The listing builds one solid part. Answer for the finished solid, in the listing's coordinates (mm). A direction names the side the tool comes from. Round coordinates to 2 decimals unless told otherwise and drop trailing zeros. Order: outer loops, then holes, each group sorted by start corner. A loop starts at its lowest first (then second) coordinate and runs counter-clockwise, first axis right, second up. Notation, with made-up numbers: M -6.75,77.25 L 6.25,77.25 A19 cw 6.25,100.25 Z; hole C 62.25,52.5 d5. An arc over 180 degrees is marked long. Write item = value, one per line. Start each with the question number.
(1) Which of the six approach directions +Z, -Z, +X, -X, +Y, -Y give full straight-line access (tool end or side, diameter ignored) to faces 1 (the face through (7.45, 0, -43)), 2 (the face through (8.72, -0.1, 51.9)), 3 (the face through (10.7, 0, 37)), 4 (the face through (6.7, 0, -46)), 5 (the face through (-4.3, 0, 37))?
(2) Each of these flat-tipped pins is pushed along its axis until it touches: pin 1 (4.5 mm diameter, centred on y = 3, z = -43.5, fed in from +X); pin 2 (3 mm diameter, centred on x = 9, y = -0.5, fed in from +Z); pin 3 (0.9 mm diameter, centred on y = 3, z = 55.5, fed in from +X); pin 4 (1.5 mm diameter, centred on x = 1.5, z = -36, fed in from -Y). Where does it stop, or does it pass through?
(3) A cutting plane is placed at B-B, the plane z = -0.5. Determine the outline of the cut face in (x, y), and give its area (3 significant figures).
(4) For a pull along Z with two mould halves and no side action, classify faces 6 (the face through (12.55, -0.1, 43.48)), 7 (the face through (-6.4, 0.1, -8.5)), 8 (the face through (10.2, 0, -43)) as released by +Z, released by -Z, zero draft, split by the parting line, or undercut.
(5) A cutting plane is placed at A-A, the plane x = 3.5. Determine the outline of the cut face in (y, z) (3 decimals).
(6) A cutting plane is placed at C-C, the plane x = -1.25. Determine the outline of the cut face in (y, z) (3 decimals).
(7) Straight lines are drawn through the part: probe 1 along Z at (x, y) = (3.25, -0.75) (3 decimals); probe 2 along X at (y, z) = (5.25, -1); probe 3 along X at (y, z) = (-4, -40). For each, find the intervals that lie inside material, in ascending order. Write a range as from..to.
from build123d import *

# Parameters (mm, degrees)
F1_DEPTH = 7.45
F2_W     = 9.95
F2_H     = 59.4720471648
F3_DEPTH = 14.901
F5_DEPTH = 14.9


with BuildPart() as f1:
    # F0 (on Front) → F1 (new body, symmetric)
    with BuildSketch(Plane.XZ):
        with BuildLine():
            Line((-8.5, -30.0970471648), (-4.3, -36.825))
            Line((-4.3, -36.825), (-4.3, -40.625))
            ThreePointArc((-4.3, -40.625), (-4.0071067812, -41.3321067812), (-3.3, -41.625))
            Line((-3.3, -41.625), (7.45, -41.625))
            Line((7.45, -41.625), (7.45, -44.825))
            Line((7.45, -44.825), (6.7, -44.825))
            Line((6.7, -44.825), (6.7, -47.025))
            Line((6.7, -47.025), (10.2, -47.025))
            Line((10.2, -47.025), (10.2, -38.425))
            ThreePointArc((10.2, -38.425), (9.9071067812, -37.7178932188), (9.2, -37.425))
            Line((9.2, -37.425), (0, -37.425))
            Line((0, -37.425), (0, 37.425))
            Line((0, 37.425), (8.4, 37.425))
            Line((8.4, 37.425), (8.4, 33.425))
            ThreePointArc((8.4, 33.425), (8.6928932188, 32.7178932188), (9.4, 32.425))
            Line((9.4, 32.425), (9.7, 32.425))
            ThreePointArc((9.7, 32.425), (10.4071067812, 32.7178932188), (10.7, 33.425))
            Line((10.7, 33.425), (10.7, 40.875))
            Line((10.7, 40.875), (12.0584372697, 42.3947607825))
            ThreePointArc((12.0584372697, 42.3947607825), (12.5542284753, 43.4993517405), (12.3218441058, 44.6875973417))
            Line((12.3218441058, 44.6875973417), (9.6272657122, 49.6124442137))
            ThreePointArc((9.6272657122, 49.6124442137), (8.7116734449, 51.9351925206), (8.4, 54.4123539124))
            Line((8.4, 54.4123539124), (8.4, 57.375))
            ThreePointArc((8.4, 57.375), (8.1071067812, 58.0821067812), (7.4, 58.375))
            Line((7.4, 58.375), (7.1, 58.375))
            ThreePointArc((7.1, 58.375), (6.3928932188, 58.0821067812), (6.1, 57.375))
            Line((6.1, 57.375), (6.1, 54.4123539124))
            ThreePointArc((6.1, 54.4123539124), (6.4116734449, 51.9351925206), (7.3272657122, 49.6124442137))
            Line((7.3272657122, 49.6124442137), (10.0218441058, 44.6875973417))
            ThreePointArc((10.0218441058, 44.6875973417), (10.2542284753, 43.4993517405), (9.7584372697, 42.3947607825))
            Line((9.7584372697, 42.3947607825), (8.4, 40.875))
            Line((8.4, 40.875), (-3.3, 40.875))
            ThreePointArc((-3.3, 40.875), (-4.0071067812, 40.5821067812), (-4.3, 39.875))
            Line((-4.3, 39.875), (-4.3, 33.875))
            Line((-4.3, 33.875), (-8.5, 29.375))
            Line((-8.5, 29.375), (-8.5, 20.075))
            Line((-8.5, 20.075), (-13.95, 20.075))
            Line((-13.95, 20.075), (-13.95, 29.375))
            Line((-13.95, 29.375), (-16.45, 29.375))
            ThreePointArc((-16.45, 29.375), (-17.8642135624, 28.7892135624), (-18.45, 27.375))
            Line((-18.45, 27.375), (-18.45, 13.875))
            Line((-18.45, 13.875), (-8.5, 6.6029528352))
            Line((-8.5, 6.6029528352), (-8.5, -30.0970471648))
        make_face()
    extrude(amount=F1_DEPTH, both=True)

    # F2 (on face) → F3 (cut, through all)
    with BuildSketch(Plane.XZ.offset(7.45)):
        with Locations((-13.475, -0.3610235824)):
            Rectangle(F2_W, F2_H)
    extrude(amount=-F3_DEPTH, mode=Mode.SUBTRACT)

    # F4 (on face) → F5 (cut, through all)
    with BuildSketch(Plane(origin=(0, 7.45, 0), x_dir=(-1, 0, 0), z_dir=(0, 1, 0))):
        Polygon((10, -4.6428571429), (10, 4.6428571429), (4.3, 10.75), (4.3, 0), (4.3, -10.75), align=None)
    extrude(amount=-F5_DEPTH, mode=Mode.SUBTRACT)


solid = f1.part
Reported:
q1.face_1 = -X, +Y, -Y
q1.face_2 = +Z, +X, +Y, -Y
q1.face_3 = -Z, +X, +Y, -Y
q1.face_4 = -Z, -X, +Y, -Y
q1.face_5 = +Z, -X, +Y, -Y
q2.pin_1 = 10.2
q2.pin_2 = 58.37
q2.pin_3 = 8.4
q2.pin_4 = through
q3.outline = M -4.3,-7.45 L 0,-7.45 L 0,7.45 L -4.3,7.45 Z
q3.area = 64.1 mm²
q4.face_6 = split by the parting line
q4.face_7 = undercut
q4.face_8 = zero draft
q5.outline = M -7.45,-41.625 L 7.45,-41.625 L 7.45,-37.425 L -7.45,-37.425 Z; M -7.45,37.425 L 7.45,37.425 L 7.45,40.875 L -7.45,40.875 Z
q6.outline = M -7.45,-41.625 L 7.45,-41.625 L 7.45,40.875 L -7.45,40.875 Z
q7.probe_1 = -41.625..-37.425, 37.425..40.875
q7.probe_2 = -4.3..0
q7.probe_3 = -4.3..10.2
